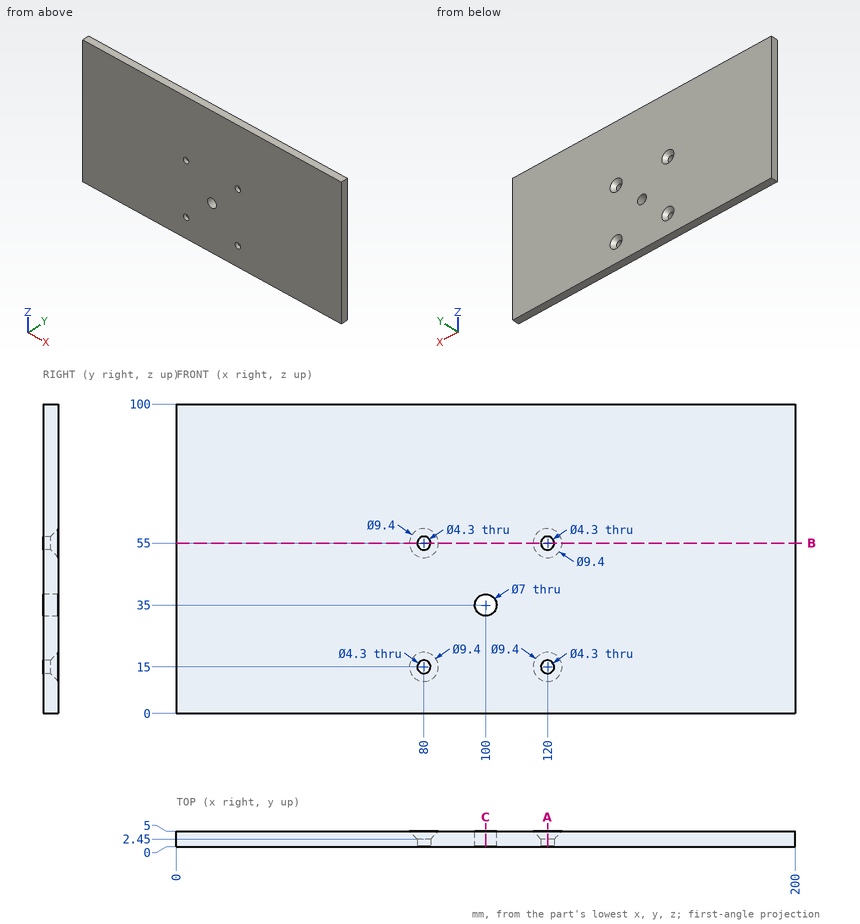
For this review, use the dimensioned drawing (mm, ordinates from the lowest corner) and the shaded views. Coordinates: 2 decimals unless noted, no trailing zeros. Loops run counter-clockwise (first coordinate to the right, second up) from the corner with the lowest first, then second, coordinate; pieces in that order, holes last.
1. Add section C-C, the plane x = 100. Give the boundary of the cut face in (y, z), then the cut area to 3 significant figures.
2. Insertion check: P1, Ø5, axis at x = 80, z = 55, coming from the +Y side. The pin has a flat end and moves straight along its axis. Give the tip position at first contact, or say it passes through.
3. Add section A-A, the plane x = 120. Give the boundary of the cut face in (y, z), then the cut area to 3 significant figures.
4. Add section B-B, the plane z = 55. Give the boundary of the cut face in (x, y).
5. For line 1 (X direction, y = 0.7, z = 55); line 2 (X direction, y = 3.8, z = 52); line 3 (Z direction, x = 98, y = 0.95), list the stretches that pass through material, from the lowest coordinate up.
Result:
1. outline: (0, 0) - (5, 0) - (5, 31.5) - (0, 31.5) - close; (0, 38.5) - (5, 38.5) - (5, 100) - (0, 100) - close
1. area: 465 mm2
2. P1: stops at y = 2.8
3. outline: (0, 0) - (5, 0) - (5, 10.3) - (2.45, 12.85) - (0, 12.85) - close; (0, 17.15) - (2.45, 17.15) - (5, 19.7) - (5, 50.3) - (2.45, 52.85) - (0, 52.85) - close; (0, 57.15) - (2.45, 57.15) - (5, 59.7) - (5, 100) - (0, 100) - close
3. area: 444 mm2
4. outline: (0, 0) - (77.85, 0) - (77.85, 2.45) - (75.3, 5) - (0, 5) - close; (82.15, 0) - (117.85, 0) - (117.85, 2.45) - (115.3, 5) - (84.7, 5) - (82.15, 2.45) - close; (122.15, 0) - (200, 0) - (200, 5) - (124.7, 5) - (122.15, 2.45) - close
5. line 1: x = 0 to 77.85, 82.15 to 117.85, 122.15 to 200
5. line 2: x = 0 to 78.2, 81.8 to 118.2, 121.8 to 200
5. line 3: z = 0 to 32.13, 37.87 to 100
